Autodesk Fusion 360 part; units mm, degrees
sketch "Sketch1" plane through (0, 0, 0) normal (0, 0, 1) x (1, 0, 0)
  line L0 (10, 27.85) -> (-10, 27.85)
  line L1 (-10, 27.85) -> (-10, -27.85)
  line L2 (-10, -27.85) -> (10, -27.85)
  line L3 (10, -27.85) -> (10, 27.85)
  line L4 (10, 27.85) -> (-10, -27.85) construction
  line L5 (-10, 27.85) -> (10, -27.85) construction
  line L6 (-10, 0) -> (-17.5, 0) construction
  line L7 (10, 0) -> (17.5, 0) construction
  line L8 (0, 27.85) -> (0, 35.85) construction
  line L9 (0, -27.85) -> (0, -35.85) construction
  line L10 (17.5, 0) -> (17.5, 35.85)
  line L11 (0, 35.85) -> (17.5, 35.85)
  line L12 (17.5, 35.85) -> (-17.5, 35.85)
  line L13 (-17.5, 35.85) -> (-17.5, -35.85)
  line L14 (-17.5, -35.85) -> (17.5, -35.85)
  line L15 (17.5, -35.85) -> (17.5, 35.85)
  line L16 (-17.5, 35.85) -> (-32.5, 35.85)
  line L17 (-32.5, 35.85) -> (-32.5, 28.35)
  line L18 (-32.5, 28.35) -> (-17.5, 28.35)
  line L19 (-17.5, -35.85) -> (-32.5, -35.85)
  line L20 (-32.5, -35.85) -> (-32.5, -28.35)
  line L21 (-32.5, -28.35) -> (-17.5, -28.35)
  circle A0 centre (-32.5, 32.1) radius 3.75
  circle A1 centre (-32.5, -32.1) radius 3.75
  dimension "d1" = 20
  dimension "d2" = 55.7
  dimension "d3" = 7.5
  dimension "d4" = 7.5
  dimension "d5" = 8
  dimension "d6" = 8
  dimension "d7" = 35
  dimension "d8" = 15
  dimension "d9" = 7.5
  dimension "d10" = 15
  dimension "d11" = 7.5
extrude "Extrude1" add sketch "Sketch1" along normal blind 8.75
sketch "Sketch2" plane through (0, 0, 8.75) normal (0, 0, 1) x (-1, 0, 0)
  line L0 (-10, -27.85) -> (-10, 27.85)
  line L1 (-10, 27.85) -> (10, 27.85)
  line L2 (10, 27.85) -> (10, -27.85)
  line L3 (10, -27.85) -> (-10, -27.85)
  line L4 (32.5, 35.85) -> (-17.5, 35.85)
  line L5 (-17.5, 35.85) -> (-17.5, -35.85)
  line L6 (-17.5, -35.85) -> (32.5, -35.85)
  arc A0 (32.5, -35.85) -> (32.5, -28.35) centre (32.5, -32.1) ccw
  line L7 (32.5, -28.35) -> (17.5, -28.35)
  line L8 (17.5, -28.35) -> (17.5, 28.35)
  line L9 (17.5, 28.35) -> (32.5, 28.35)
  arc A1 (32.5, 28.35) -> (32.5, 35.85) centre (32.5, 32.1) ccw
  circle A2 centre (32.5, -32.1) radius 2.925
  circle A3 centre (32.5, 32.1) radius 2.925
  circle A4 centre (32.5, -32.1) radius 1.875
  circle A5 centre (32.5, 32.1) radius 1.875
  line L10 (17.5, 0) -> (10, 0) construction
  line L11 (-10, 0) -> (-17.5, 0) construction
  circle A6 centre (13.75, 0) radius 2.925
  circle A7 centre (13.75, 0) radius 1.875
  circle A8 centre (-13.75, 0) radius 2.925
  circle A9 centre (-13.75, 0) radius 1.875
  dimension "d14" = 5.85
  dimension "d15" = 5.85
  dimension "d16" = 3.75
  dimension "d17" = 3.75
  dimension "d18" = 5.85
  dimension "d19" = 3.75
  dimension "d20" = 5.85
  dimension "d21" = 3.75
extrude "Extrude2" cut sketch "Sketch2" against normal blind 26 contours A4 | A5 | A7 | A9
extrude "Extrude3" cut sketch "Sketch2" against normal blind 3.1 contours A2 | A3 | A6 | A8
fillet "Fillet1" radius 7.5 2 edges at (17.5, 35.85, 4.375) (17.5, -35.85, 4.375)
Design review of the part built by this model. Coordinates are the model's own, in mm. A direction names the side the tool comes from. Give positions to 0.01 mm unless a question says otherwise; leave off trailing zeros. Order: outer loops, then holes, each group sorted by start corner. A loop starts at its lowest first (then second) coordinate and runs counter-clockwise, first axis right, second up. Notation, with made-up numbers: (37, 68) - (86, 68) arc R28 ccw to (86, 106) - close; hole circle Ø5 at (64, 66.5). An arc over 180 degrees is marked (long way). Use CSV: the item, a comma, the result in double quotes. Start each with the question number.
Q1. Draft analysis for pull direction Y (two halves, no side actions). For faces 1 (the face through (17.5, 0, 4)), 2 (the face through (-12, 35.85, 4)), 3 (the face through (-15.54, -0.56, 2.86)), state which applies: pulls with the +Y half, pulls with the -Y half, needs draft (parallel to the pull), parting line crosses it, or undercut.
Q2. Take a section at D-D (x = 13.75). State the section outline as (y, z) points (3 decimals), and give its area (3 significant figures).
Q3. Take a section at A-A (x = -13.75). State the section outline as (y, z) points (3 decimals).
Q4. Take a section at B-B (z = 7.75). State the section outline as (x, y) points (3 decimals), and give its area (3 significant figures).
Q5. For P1, Ø3.5, axis at x = -32.5, y = -32.1, coming from the -Z side; P2, Ø2, axis at y = -19.5, z = 2, coming from the -X side; P3, Ø5, axis at y = 28, z = 7.5, coming from the -X side, all flat-tipped, find the tip position at first contact; note any pin that passes through.
Q6. Machinability: for faces 4 (the face through (0, -27.85, 4)), 5 (the face through (-25, 28.35, 4)), 6 (the face through (13, 2, 5.65)), which of the approach directions +Z, -Z, +X, -X, +Y, -Y give a long, thin tool a straight path to every point of the face, cutting with its end or side? Answer none if there is none.
Q7. For line 1 (X direction, y = 0, z = 6.35) (3 decimals); line 2 (Y direction, x = -32.5, z = 8.1) (3 decimals); line 3 (X direction, y = 0, z = 3) (3 decimals), list the stretches that pass through material, from the lowest coordinate up.
Q8. Take a section at C-C (y = 8). State the section outline as (x, z) points, and give its area (3 significant figures).
Calculated:
1,face 1,"needs draft"
1,face 2,"pulls with the +Y half"
1,face 3,"undercut"
2,outline,"(-34.845, 0) - (-1.875, 0) - (-1.875, 5.65) - (-2.925, 5.65) - (-2.925, 8.75) - (-34.845, 8.75) - close; (1.875, 0) - (34.845, 0) - (34.845, 8.75) - (2.925, 8.75) - (2.925, 5.65) - (1.875, 5.65) - close"
2,area,"570 mm²"
3,outline,"(-35.85, 0) - (-1.875, 0) - (-1.875, 5.65) - (-2.925, 5.65) - (-2.925, 8.75) - (-35.85, 8.75) - close; (1.875, 0) - (35.85, 0) - (35.85, 8.75) - (2.925, 8.75) - (2.925, 5.65) - (1.875, 5.65) - close"
4,outline,"(-32.5, -35.85) - (10, -35.85) arc R7.5 ccw to (17.5, -28.35) - (17.5, 28.35) arc R7.5 ccw to (10, 35.85) - (-32.5, 35.85) arc R3.75 ccw to (-32.5, 28.35) - (-17.5, 28.35) - (-17.5, -28.35) - (-32.5, -28.35) arc R3.75 ccw to start; hole circle Ø5.85 at (-32.5, -32.1); hole circle Ø5.85 at (-32.5, 32.1); hole circle Ø5.85 at (-13.75, 0); hole (-10, -27.85) - (10, -27.85) - (10, 27.85) - (-10, 27.85) - close; hole circle Ø5.85 at (13.75, 0)"
4,area,"1,530 mm²"
5,P1,"passes through"
5,P2,"stops at x = -17.5"
5,P3,"stops at x = -35.89"
6,face 4,"+Z, -Z"
6,face 5,"+Z, -Z, -X"
6,face 6,"+Z"
7,line 1,"x = -17.5 to -16.675, -10.825 to -10, 10 to 10.825, 16.675 to 17.5"
7,line 2,"y = -35.85 to -35.025, -29.175 to -28.35, 28.35 to 29.175, 35.025 to 35.85"
7,line 3,"x = -17.5 to -15.625, -11.875 to -10, 10 to 11.875, 15.625 to 17.5"
8,outline,"(-17.5, 0) - (-10, 0) - (-10, 8.75) - (-17.5, 8.75) - close; (10, 0) - (17.5, 0) - (17.5, 8.75) - (10, 8.75) - close"
8,area,"131 mm²"
